Input: dimensioned drawing with shaded views. Units: mm. Origin: part minimum x, y, z. Coordinates: 2 decimals unless noted, no trailing zeros. Loops run counter-clockwise (first coordinate to the right, second up) from the corner with the lowest first, then second, coordinate; pieces in that order, holes last. Notation, with made-up numbers: (-21.5, 27.25) - (35.5, 27.25) arc R29 cw to (35.5, 55.25) - close; hole circle Ø4 at (7, 42.5). An arc over 180 degrees is marked (long way). Use one line per item in the form item = value. Start each with the question number.
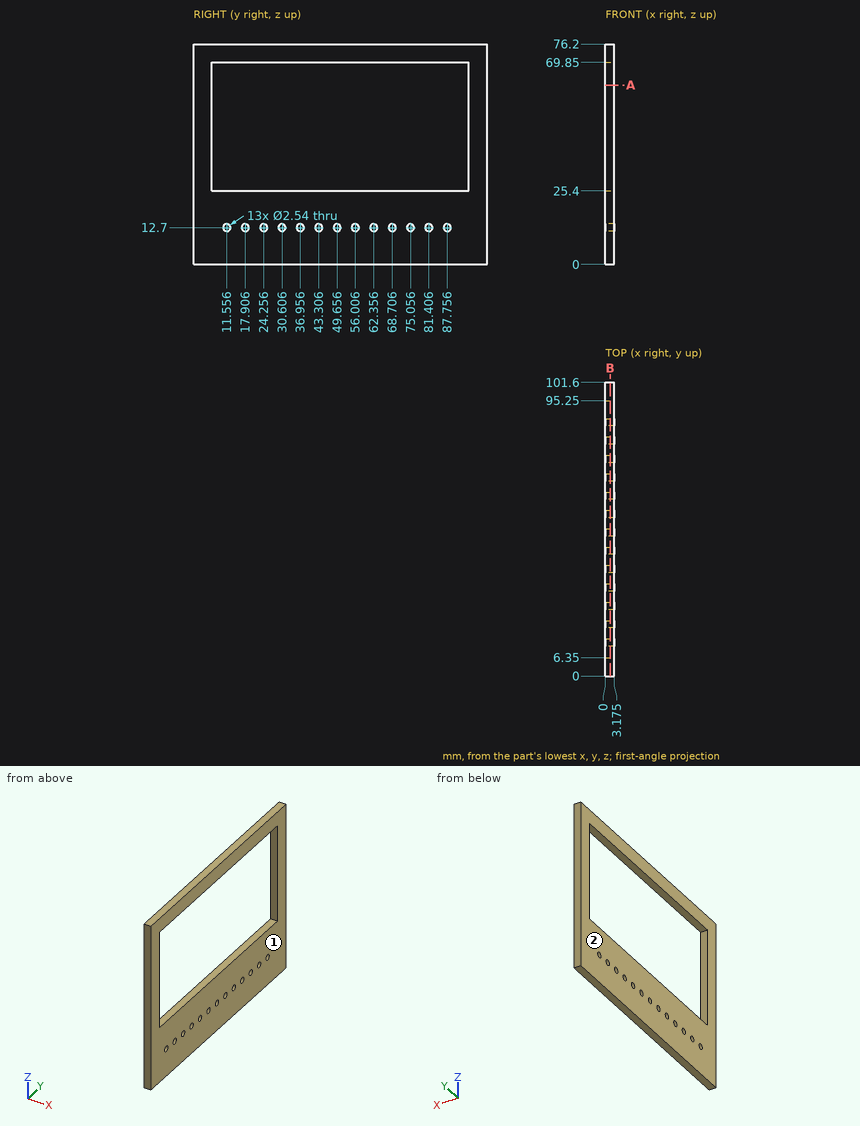
(1) Mould query, pull axis X, two halves, no side actions, for the marked faces 1 and 2. Classes: +X half, -X half, draft (parallel to the pull), parting line (faces both ways), or undercut.
(2) Cut plane A-A, the plane z = 62. Output: boundary loops of the cut face in (x, y) (3 decimals), plus the area to 3 significant figures.
(3) Material intervals for line 1 (Z direction, x = 0.25, y = 90); line 2 (Y direction, x = 0.75, z = 46.5); line 3 (Z direction, x = 2.35, y = 43), sorted ascending.
(4) Cut plane B-B, the plane x = 1.65. State how many separate pieces and enclosed holes the cut face has, plus the area to 3 significant figures.
(5) Contact query for flat-ended pins moving along their axis: pin 1 (3 mm diameter, centred on y = 36.96, z = 12.7, fed in from +X) (3 decimals); pin 2 (1.5 mm diameter, centred on y = 11.56, z = 12.7, fed in from +X). Output: stop coordinate, or through.
Recorded:
q1.face_1 = +X half
q1.face_2 = -X half
q2.outline = (0, 0) - (3.175, 0) - (3.175, 6.35) - (0, 6.35) - close; (0, 95.25) - (3.175, 95.25) - (3.175, 101.6) - (0, 101.6) - close
q2.area = 40.3 mm²
q3.line_1 = 0 to 25.4, 69.85 to 76.2
q3.line_2 = 0 to 6.35, 95.25 to 101.6
q3.line_3 = 0 to 11.47, 13.93 to 25.4, 69.85 to 76.2
q4.separate_pieces = 1
q4.enclosed_holes = 14
q4.area = 3,720 mm²
q5.pin_1 = 3.175
q5.pin_2 = through
